Build history of the part. All positions in model axes, mm. Face numbers are marked on the shaded views. A direction names the side the tool comes from. Round coordinates to 2 decimals unless told otherwise and drop trailing zeros. Order: outer loops, then holes, each group sorted by start corner. A loop starts at its lowest first (then second) coordinate and runs counter-clockwise, first axis right, second up. Notation, with made-up numbers: (67, 75.25) -> (93, 75.25) arc R21 ccw to (93, 112.25) -> close; hole circle Ø4 at (68.25, 67.5). An arc over 180 degrees is marked (long way). Answer as a JSON object with one key per item and string values.
Autodesk Inventor part; units mm, degrees
ref_plane "YZ Plane" through (0, 0, 0) normal (1, 0, 0) x (0, 1, 0)
ref_plane "XZ Plane" through (0, 0, 0) normal (0, 1, 0) x (-1, 0, 0)
ref_plane "XY Plane" through (0, 0, 0) normal (0, 0, 1) x (1, 0, 0)
sketch "Skizze1" plane through (0, 0, 0) normal (0, 1, 0) x (-1, 0, 0)
  circle A0 centre (0, 0) radius 15
  dimension "d0" = 30
extrude "Extrusion1" add sketch "Skizze1" along normal blind 10
sketch "Skizze2" plane through (0, 0, 0) normal (0, -1, 0) x (1, 0, 0)
  line L0 (14.3188, 0.9) -> (12.9688, 0.9)
  line L1 (12.9688, -0.9) -> (14.3188, -0.9)
  line L2 (14.3188, -0.9) -> (14.3188, 0.9)
  line L3 (-21.3175, 0) -> (21.3175, 0)
  arc A0 (12.9688, 0.9) -> (0.9, 12.9688) centre (0, 0) ccw
  line L4 (-0.9, -12.9688) -> (-0.9, -14.3188)
  line L5 (-0.9, -14.3188) -> (0.9, -14.3188)
  line L6 (0.9, -14.3188) -> (0.9, -12.9688)
  line L7 (-12.9688, 0.9) -> (-14.3188, 0.9)
  line L8 (-14.3188, 0.9) -> (-14.3188, -0.9)
  line L9 (-14.3188, -0.9) -> (-12.9688, -0.9)
  line L10 (-0.9, 12.9688) -> (-0.9, 14.3188)
  line L11 (-0.9, 14.3188) -> (0.9, 14.3188)
  line L12 (0.9, 14.3188) -> (0.9, 12.9688)
  line L13 (0, -21.3175) -> (0, 21.3175)
  line L14 (-21.3175, 0) -> (21.3175, 0)
  arc A1 (0.9, -12.9688) -> (12.9688, -0.9) centre (0, 0) ccw
  arc A2 (-12.9688, -0.9) -> (-0.9, -12.9688) centre (0, 0) ccw
  arc A3 (-0.9, 12.9688) -> (-12.9688, 0.9) centre (0, 0) ccw
  circle A4 centre (0, 0) radius 4.2
  circle A5 centre (7, 7.1414) radius 1.2
  circle A6 centre (-5.6, -5.7131) radius 1.2
  dimension "d4" = 0.9
  dimension "d5" = 0.9
  dimension "d8" = 1.35
  dimension "d9" = 1.35
  dimension "d10" = 1.8
  dimension "d11" = 0.9
  dimension "d12" = 1.35
  dimension "d13" = 1.8
  dimension "d14" = 0.9
  dimension "d15" = 0.9
  dimension "d16" = 1.35
  dimension "d17" = 8.4
  dimension "d18" = 2.4
  dimension "d19" = 2.4
  dimension "d20" = 8
  dimension "d21" = 10
  dimension "d22" = 7
  dimension "d23" = 5.6
  dimension "d50" = 13
  dimension "d51" = 13
  dimension "d52" = 1.35
  dimension "d53" = 1.35
  dimension "d54" = 1.35
extrude "Extrusion2" cut sketch "Skizze2" against normal blind 3 contours L2 L3 A4 L13 L11 L12 A0 L0 | L2 L1 A1 L6 L5 L13 A4 L3 | A4 L3 L8 L7 A3 L10 L11 L13 | L13 L5 L4 A2 L9 L8 L3 A4
sketch "Skizze4" plane through (7, 0, 7.1414) normal (0, -1, 0) x (1, 0, 0)
  circle A0 centre (-7, -7.1414) radius 4.2
  circle A1 centre (-12.6, -12.8546) radius 1.2
  circle A2 centre (0, 0) radius 1.2
  line L0 (-7, -28.1414) -> (-7, 13.8586)
  dimension "d26" = 2.4
  dimension "d27" = 5.6
  dimension "d28" = 8
  dimension "d44" = 8.4
  dimension "d45" = 2.4
extrude "Extrusion3" add sketch "Skizze4" along normal blind 2
sketch "Skizze5" plane through (0, 10, 0) normal (0, 1, 0) x (1, 0, 0)
  circle A0 centre (0, 0) radius 19.262
  circle A1 centre (0, 0) radius 7
  dimension "d31" = 14
extrude "Extrusion4" cut sketch "Skizze5" against normal blind 7
fillet "Rundung1" radius 1 8 edges at (12.9688, 1.5, -0.9) (12.9688, 1.5, 0.9) (0.9, 1.5, -12.9688) (-0.9, 1.5, -12.9688) (-12.9688, 1.5, -0.9) (-12.9688, 1.5, 0.9) (-0.9, 1.5, 12.9688) (0.9, 1.5, 12.9688)
sketch "Skizze8" plane through (0, 10, 0) normal (0, 1, 0) x (1, 0, 0)
  circle A0 centre (0, 0) radius 1
  dimension "d46" = 2
extrude "Extrusion7" cut sketch "Skizze8" against normal blind 7
sketch "Skizze9" plane through (0, -2, 0) normal (0, -1, 0) x (1, 0, 0)
  line L0 (18.2687, 9.2162) -> (-7.478, -18.1772)
  line L1 (-7.478, -18.1772) -> (18.2687, -18.1772)
  line L2 (18.2687, -18.1772) -> (18.2687, 9.2162)
  line L3 (8.0673, 18.8043) -> (-17.6793, -8.5891)
  line L4 (-17.6793, -8.5891) -> (-17.6793, 18.8043)
  line L5 (-17.6793, 18.8043) -> (8.0673, 18.8043)
  point P0 (0, 0)
  dimension "d55" = 7
  dimension "d56" = 7
extrude "Extrusion8" cut sketch "Skizze9" against normal blind 50
sketch "Skizze10" plane through (0, -2, 0) normal (0, -1, 0) x (1, 0, 0)
  circle A0 centre (0, 0) radius 11.5
  circle A1 centre (0, 0) radius 18.9246
  dimension "d61" = 23
extrude "Extrusion9" cut sketch "Skizze10" against normal blind 10
sketch "Skizze11" plane through (0, -2, 0) normal (0, -1, 0) x (1, 0, 0)
  circle A0 centre (0, 0) radius 1
  circle A1 centre (0, 0) radius 4.2
extrude "Extrusion10" cut sketch "Skizze11" against normal blind 8.5 contours A0 | A1
sketch "Skizze13" plane through (0, 3, 0) normal (0, -1, 0) x (1, 0, 0)
  circle A0 centre (7, 7.1414) radius 1.2
  circle A1 centre (7, 7.1414) radius 1.2
  circle A2 centre (-5.6, -5.7131) radius 1.2
  circle A3 centre (-5.6, -5.7131) radius 1.2
  arc A4 (11.3495, 1.8544) -> (1.1481, 11.4425) centre (0, 0) ccw
  line L0 (11.3495, 1.8544) -> (8.9749, -0.6721)
  line L1 (11.3495, 1.8544) -> (-1.1481, -11.4425)
  line L2 (1.1481, 11.4425) -> (-11.3495, -1.8544)
  line L3 (1.2265, -8.916) -> (-1.1481, -11.4425)
  arc A5 (-11.3495, -1.8544) -> (-1.1481, -11.4425) centre (0, 0) ccw
  circle A6 centre (0, 0) radius 4.2
extrude "Extrusion11" add sketch "Skizze13" along normal blind 3.5
sketch "Skizze14" plane through (7, -2, 7.1414) normal (0, -1, 0) x (1, 0, 0)
  circle A0 centre (0, 0) radius 1.2
  circle A1 centre (0, 0) radius 1.2
  circle A2 centre (-12.6, -12.8546) radius 1.2
  circle A3 centre (-12.6, -12.8546) radius 1.2
  point P0 (-7, -7.1414)
extrude "Extrusion12" add sketch "Skizze14" along normal blind 0.5
sketch "Skizze15" plane through (0, 10, 0) normal (0, 1, 0) x (1, 0, 0)
  circle A0 centre (0, 0) radius 1
  circle A1 centre (0, 0) radius 2.35
  dimension "d68" = 4.7
extrude "Extrusion13" cut sketch "Skizze15" against normal blind 3.3 contours A0 | A1
sketch "Skizze17" plane through (0, -0.5, 0) normal (0, -1, 0) x (1, 0, 0)
  line L0 (2.8954, 11.8415) -> (-13.3125, -5.4031)
  line L1 (1.1481, 11.4425) -> (-5.1007, 4.7941)
  line L2 (-13.3125, -5.4031) -> (-13.3125, 19.7684)
  line L3 (-13.3125, 19.7684) -> (2.8954, 11.8415)
  line L4 (-3.5303, -12.5169) -> (12.8557, 4.9171)
  line L5 (-1.1481, -11.4425) -> (5.1007, -4.7941)
  line L6 (12.8557, 4.9171) -> (12.8557, -12.5169)
  line L7 (12.8557, -12.5169) -> (-3.5303, -12.5169)
  point P0 (0, 0)
  dimension "d71" = 1
  dimension "d72" = 1
extrude "Extrusion14" cut sketch "Skizze17" against normal blind 15
properties part number "Adaptation_on_OPdevside_4_3"
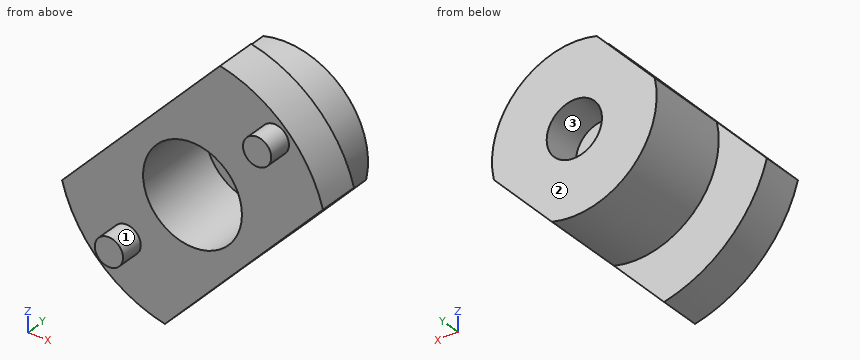
1) Cut at D-D, the plane x = -5.6. Give the cut face in (y, z).
Checked values:
{"outline": "(-2.5, -6.91) -> (-0.5, -6.91) -> (-0.5, -10.04) -> (3, -10.04) -> (3, -4.2) -> (10, -4.2) -> (10, 2.8) -> (-0.5, 2.8) -> (-0.5, -4.51) -> (-2.5, -4.51) -> close"}
2) Cut at C-C, the plane z = 0. Give the cut face in (x, y), plus the area to 3 significant figures.
Checked values:
{"outline": "(-8.23, -0.5) -> (-4.2, -0.5) -> (-4.2, 6.5) -> (-1, 6.5) -> (-1, 6.7) -> (-2.35, 6.7) -> (-2.35, 10) -> (-7, 10) -> (-7, 3) -> (-8.23, 3) -> close; (1, 6.5) -> (4.2, 6.5) -> (4.2, -0.5) -> (8.23, -0.5) -> (8.23, 3) -> (7, 3) -> (7, 10) -> (2.35, 10) -> (2.35, 6.7) -> (1, 6.7) -> close", "area": "80.9 mm²"}
3) Flat gauge pins, fed straight in: pin 1 Ø1 at (y, z) = (6, 3) entering from -X; pin 2 Ø5 at (x, y) = (7.5, 8) entering from -Z; pin 3 Ø4 at (x, z) = (0, 0) entering from -Y. Where does each tip first touch, or does it go through?
Checked values:
{"pin 1": "stops at x = -5.88", "pin 2": "stops at z = -3.44", "pin 3": "stops at y = 6.5"}
4) Which spindle directions (+Z, -Z, +X, -X, +Y, -Y) get a long thin tool onto all of the face, cutting with end or side? Do the marked faces 1, 2 and 3. Say none if no direction does.
Checked values:
{"face 1": "-Y", "face 2": "+Z, -Z, +X, -X, +Y", "face 3": "+Y"}
5) Cut at A-A, the plane y = 2.5. Give the cut face in (x, z).
Checked values:
{"outline": "(-11.09, -3.04) arc R11.5 ccw to (-2.35, -11.26) -> (11.09, 3.04) arc R11.5 ccw to (2.35, 11.26) -> close; hole circle Ø8.4 at (0, 0)"}
6) Cut at B-B, the plane x = 0. Give the cut face in (y, z).
Checked values:
{"outline": "(-0.5, -8.76) -> (3, -8.76) -> (3, -7) -> (10, -7) -> (10, -2.35) -> (6.7, -2.35) -> (6.7, -1) -> (6.5, -1) -> (6.5, -4.2) -> (-0.5, -4.2) -> close; (-0.5, 4.2) -> (6.5, 4.2) -> (6.5, 1) -> (6.7, 1) -> (6.7, 2.35) -> (10, 2.35) -> (10, 7) -> (3, 7) -> (3, 8.76) -> (-0.5, 8.76) -> close"}
7) Probe L1, parallel to Z at x = 0, y = 6.6; L2, parallel to Z at x = 0, y = 3.25; L3, parallel to X at y = 8.75, z = 0. List the from-to ranges inside material, lowest first. Write a range as from..to.
Checked values:
{"L1": "z = -7..-1, 1..7", "L2": "z = -7..-4.2, 4.2..7", "L3": "x = -7..-2.35, 2.35..7"}
